from build123d import *

# Parameters (mm, degrees)
SKETCH7_W           = 80
SKETCH7_H           = 120
BOSS_EXTRUDE2_DEPTH = 10
SKETCH8_W           = 78
SKETCH8_H           = 18
CUT_EXTRUDE1_DEPTH  = 2
SKETCH9_W           = 18
SKETCH9_H           = 117
CUT_EXTRUDE2_DEPTH  = 2
SKETCH10_W          = 78
SKETCH10_H          = 18
CUT_EXTRUDE3_DEPTH  = 2
FILLET1_R           = 2


with BuildPart() as part:
    # Sketch7 → Boss-Extrude2 (new, symmetric)
    with BuildSketch(Plane.XY):
        with Locations((38.421052632, -28.157894737)):
            Rectangle(SKETCH7_W, SKETCH7_H)
    extrude(amount=BOSS_EXTRUDE2_DEPTH, both=True)

    # Sketch8 → Cut-Extrude1 (cut)
    with BuildSketch(Plane(origin=(0, 31.842105263, 0), x_dir=(1, 0, 0), z_dir=(0, 1, 0))):
        with Locations((39.421052632, 0)):
            Rectangle(SKETCH8_W, SKETCH8_H)
    extrude(amount=-CUT_EXTRUDE1_DEPTH, mode=Mode.SUBTRACT)

    # Sketch9 → Cut-Extrude2 (cut)
    with BuildSketch(Plane(origin=(78.421052632, 0, 0), x_dir=(0, 0, -1), z_dir=(1, 0, 0))):
        with Locations((0, -28.657894737)):
            Rectangle(SKETCH9_W, SKETCH9_H)
    extrude(amount=-CUT_EXTRUDE2_DEPTH, mode=Mode.SUBTRACT)

    # Sketch10 → Cut-Extrude3 (cut)
    with BuildSketch(Plane.XZ.offset(88.157894737)):
        with Locations((39.421052632, 0)):
            Rectangle(SKETCH10_W, SKETCH10_H)
    extrude(amount=-CUT_EXTRUDE3_DEPTH, mode=Mode.SUBTRACT)

    # Fillet1
    fillet1_edges = [part.edges().sort_by_distance(p)[0] for p in [
        (-1.578947368, -28.157894737, 10),
        (-1.578947368, -28.157894737, -10),
    ]]
    fillet(fillet1_edges, radius=FILLET1_R)


solid = part.part
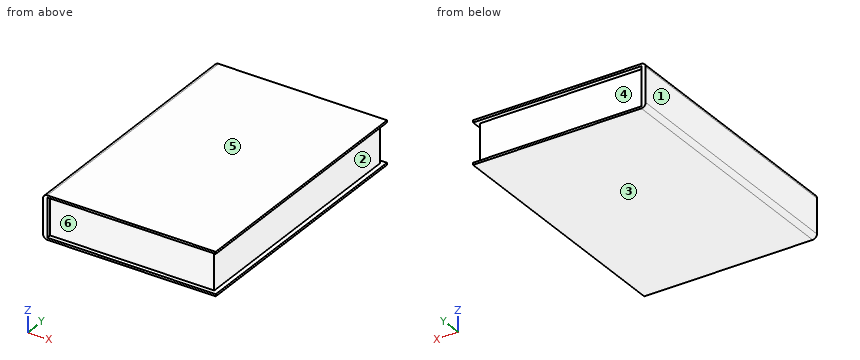
Design review of the part built by this model. Coordinates are the model's own, in mm. Face numbers are marked on the shaded views. A direction names the side the tool comes from. Coordinates: 2 decimals unless noted, no trailing zeros. Loops run counter-clockwise (first coordinate to the right, second up) from the corner with the lowest first, then second, coordinate; pieces in that order, holes last. Notation, with made-up numbers: M -5,29 L 51,29 A18 ccw 51,39 Z; hole C 74.5,-38 d3. An arc over 180 degrees is marked long. Answer as CSV lines item,"result".
Item 1: Add section C-C on y = -34. State the section outline as (x, z) points, plus the area to 3 significant figures.
Answer list:
outline,"M -1.58,-8 A2 ccw 0.42,-10 L 78.42,-10 L 78.42,-9 L 76.42,-9 L 76.42,9 L 78.42,9 L 78.42,10 L 0.42,10 A2 ccw -1.58,8 Z"
area,"1,560 mm²"
Item 2: For P1, Ø1.6, axis at y = 31, z = -1, coming from the +X side; P2, Ø12, axis at x = 62, z = 1.5, coming from the +Y side; P3, Ø9, axis at y = -31.5, z = 4, coming from the +X side, all flat-tipped, find the tip position at first contact; note any pin that passes through.
Answer list:
P1,"x = 0.42"
P2,"y = 29.84"
P3,"x = 76.42"
Item 3: Add section B-B on x = 53. State the section outline as (y, z) points, plus the area to 3 significant figures.
Answer list:
outline,"M -88.16,-10 L 31.84,-10 L 31.84,-9 L 29.84,-9 L 29.84,9 L 31.84,9 L 31.84,10 L -88.16,10 L -88.16,9 L -86.16,9 L -86.16,-9 L -88.16,-9 Z"
area,"2,330 mm²"
Item 4: The part is to be moulded in two halves that separate along Z. For the marked faces 1, 2, 3 and 4, say which applies: pulls with the +Z half, pulls with the -Z half, needs draft (parallel to the pull), parting line crosses it, or undercut.
Answer list:
face 1,"needs draft"
face 2,"undercut"
face 3,"pulls with the -Z half"
face 4,"undercut"
Item 5: For probe 1 along Y at (x, z) = (25.5, 5.75); probe 2 along X at (y, z) = (-4.5, 1); probe 3 along X at (y, z) = (21, 9.25), list the stretches that pass through material, from the lowest coordinate up.
Answer list:
probe 1,"-86.16 to 29.84"
probe 2,"-1.58 to 76.42"
probe 3,"-1.14 to 78.42"
Item 6: Machinability: for the marked faces 5 and 6, which of the approach directions +Z, -Z, +X, -X, +Y, -Y give a long, thin tool a straight path to every point of the face, cutting with its end or side? Answer none if there is none.
Answer list:
face 5,"+Z, +X, -X, +Y, -Y"
face 6,"+X, -Y"
Item 7: Add section A-A on z = 0. State the section outline as (x, y) points.
Answer list:
outline,"M -1.58,-88.16 L 0.42,-88.16 L 0.42,-86.16 L 76.42,-86.16 L 76.42,29.84 L 0.42,29.84 L 0.42,31.84 L -1.58,31.84 Z"
